from build123d import *

# Parameters (mm, degrees)
SKETCH_1_R          = 5
EXTRUDE_1_DEPTH     = 11.8
SKETCH_2_R          = 0.75
EXTRUDE_3_DEPTH     = 6.3
SKETCH_4_R          = 1
CUT_EXTRUDE_1_DEPTH = 5


with BuildPart() as part:
    # 草图1 → 凸台-拉伸1 (new body)
    with BuildSketch(Plane(origin=(0, 0, 0), x_dir=(1, 0, 0), z_dir=(0, 1, 0))):
        with Locations(Location((-0.143044278, 0, 0), (0, 0, 270))):
            Circle(SKETCH_1_R)
    extrude(amount=EXTRUDE_1_DEPTH)

    # 草图2 → 凸台-拉伸3 (add)
    with BuildSketch(Plane(origin=(0, 11.8, 0), x_dir=(1, 0, 0), z_dir=(0, 1, 0))):
        with Locations(Location((-0.143044278, 0, 0), (0, 0, 270))):
            Circle(SKETCH_2_R)
    extrude(amount=EXTRUDE_3_DEPTH)

    # 草图4 → 切除-拉伸1 (cut)
    with BuildSketch(Plane(origin=(0, 11.8, 0), x_dir=(1, 0, 0), z_dir=(0, 1, 0))):
        with Locations(Location((-0.143044278, -3.5, 0), (0, 0, 270))):
            Circle(SKETCH_4_R)
        with Locations(Location((-3.643044278, 0, 0), (0, 0, 270))):
            Circle(SKETCH_4_R)
        with Locations(Location((-0.143044278, 3.5, 0), (0, 0, 270))):
            Circle(SKETCH_4_R)
        with Locations(Location((3.356955722, 0, 0), (0, 0, 270))):
            Circle(SKETCH_4_R)
    extrude(amount=-CUT_EXTRUDE_1_DEPTH, mode=Mode.SUBTRACT)


solid = part.part
Check sheet for the modelled part. Datum: model origin and axes. Units: mm. A direction names the side the tool comes from. Coordinates: 2 decimals unless noted, no trailing zeros. Loops run counter-clockwise (first coordinate to the right, second up) from the corner with the lowest first, then second, coordinate; pieces in that order, holes last. Notation, with made-up numbers: (77, -10) -> (96, -10) arc R19 ccw to (96, -3) -> close; hole circle Ø1 at (-17, 31.5). An arc over 180 degrees is marked (long way). Write item = value, one per line. Start each with the question number.
1. Depth check by flat-ended pin: P1, Ø1, axis at x = 0, z = -3.5, coming from the +Y side; P2, Ø0.6, axis at x = 4, z = -0.5, coming from the +Y side; P3, Ø2, axis at y = 13.5, z = 2.5, coming from the +X side; P4, Ø1.5, axis at y = 2, z = -3.5, coming from the -X side. Enter the tip coordinate at first touch or a pass-through.
2. Section check B-B on y = 9. Record the cut outline in (x, z), then the cut area to 3 significant figures.
3. Tool access check on faces 1 (the cylindrical face through (-0.1, 9.3, 2.5)), 2 (the cylindrical face through (4.814, 5.817, -0.651)). Record the directions out of +Z, -Z, +X, -X, +Y, -Y that give a thin tool (end or side, any length) a straight path to the whole face; none if there is none.
4. Draft check along Z on faces 3 (the flat face through (0, 0, 0)), 4 (the cylindrical face through (-2.65, 9.34, -0.13)), 5 (the cylindrical face through (-0.43, 14.906, 0.693)). Enter one of: released by +Z, released by -Z, zero draft, split by the parting line, or undercut.
5. Material ranges on line 1 (X direction, y = 8.65, z = 0); line 2 (X direction, y = 11.25, z = -0.25); line 3 (Y direction, x = -0.25, z = -2.25), recorded low to high.
6. Section check C-C on x = -2. Record the cut outline in (y, z).
7. Section check D-D on y = 17.25. Record the cut outline in (x, z).
8. Section check A-A on z = 0. Record the cut outline in (x, y).
Responses:
q1.P1 = 6.8
q1.P2 = 11.8
q1.P3 = through
q1.P4 = -4.32
q2.outline = circle Ø10 at (-0.14, 0); hole circle Ø2 at (-3.64, 0); hole circle Ø2 at (-0.14, -3.5); hole circle Ø2 at (-0.14, 3.5); hole circle Ø2 at (3.36, 0)
q2.area = 66.0 mm2
q3.face_1 = +Y
q3.face_2 = +Y, -Y
q4.face_3 = zero draft
q4.face_4 = undercut
q4.face_5 = split by the parting line
q5.line_1 = -5.14 to -4.64, -2.64 to 2.36, 4.36 to 4.86
q5.line_2 = -5.14 to -4.61, -2.67 to 2.39, 4.33 to 4.85
q5.line_3 = 0 to 11.8
q6.outline = (0, -4.64) -> (11.8, -4.64) -> (11.8, 4.64) -> (0, 4.64) -> close
q7.outline = circle Ø1.5 at (-0.14, 0)
q8.outline = (-5.14, 0) -> (4.86, 0) -> (4.86, 11.8) -> (4.36, 11.8) -> (4.36, 6.8) -> (2.36, 6.8) -> (2.36, 11.8) -> (0.61, 11.8) -> (0.61, 18.1) -> (-0.89, 18.1) -> (-0.89, 11.8) -> (-2.64, 11.8) -> (-2.64, 6.8) -> (-4.64, 6.8) -> (-4.64, 11.8) -> (-5.14, 11.8) -> close
